Check sheet for the modelled part. Datum: model origin and axes. Units: mm. Face numbers are marked on the shaded views. A direction names the side the tool comes from. Give positions to 0.01 mm unless a question says otherwise; leave off trailing zeros. Answer as CSV lines item,"result". Start each with the question number.
(1) Section check A-A on x = 41.2. State how many separate pieces and enclosed holes the cut face has, plus the area to 3 significant figures.
(2) Material ranges on line 1 (X direction, y = -13.04, z = 2.6); line 2 (X direction, y = -12.7, z = 3.75); line 3 (Y direction, x = 41.2, z = 1.9), recorded low to high. Write a range as from..to.
(3) Access from +Z, -Z, +X, -X, +Y, -Y to the whole of each face (thin tool, end or side, straight path). Record for the marked faces 1 and 2.
(4) Gauge pin test, flat end, axial feed: pin 1 Ø5.5 at (x, y) = (41.5, -12.5) entering from +Z. Record the tip position at first contact, or that the pin passes through.
(5) Release check for a two-part mould opening along X. For the marked faces 3 and 4 record: pulls with the +X half, pulls with the -X half, needs draft (parallel to the pull), parting line crosses it, or undercut.
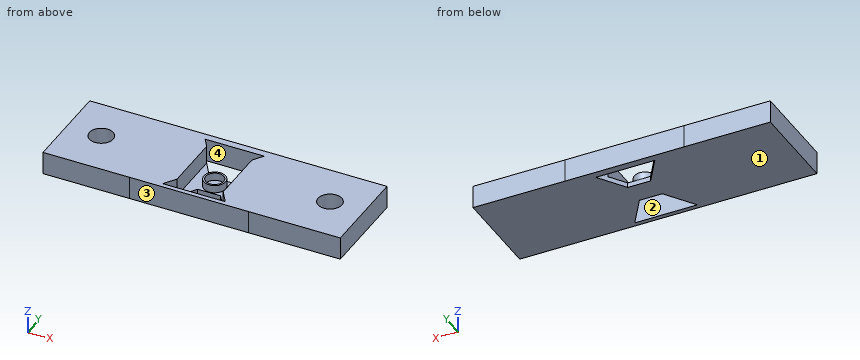
from build123d import *

# Parameters (mm, degrees)
BOX_W             = 33
BOX_H             = 2
BOX_DEPTH         = 6.35
CYLINDER001_R     = 3.302
CYLINDER001_DEPTH = 10
BOX002_W          = 12.7
BOX002_H          = 16.7
BOX002_DEPTH      = 17
CYLINDER_R        = 3.302
CYLINDER_DEPTH    = 10
EXTRUDE_DEPTH     = 6.35
CYLINDER003_R     = 2.5
CYLINDER003_DEPTH = 16
CYLINDER002_R     = 3
CYLINDER002_DEPTH = 3.5
BOX001_W          = 33
BOX001_H          = 1.25
BOX001_DEPTH      = 6.35


with BuildPart() as support1:
    # Box → Box (new body)
    with BuildSketch(Plane(origin=(24, -2.35, 0), x_dir=(1, 0, 0), z_dir=(0, 0, 1))):
        with Locations((16.5, 1)):
            Rectangle(BOX_W, BOX_H)
    extrude(amount=BOX_DEPTH)


with BuildPart() as hole2:
    # Cylinder001 → Cylinder001 (new body)
    with BuildSketch(Plane(origin=(73.025, -12.7, 1e-05), x_dir=(1, 0, 0), z_dir=(0, 0, 1))):
        Circle(CYLINDER001_R)
    extrude(amount=CYLINDER001_DEPTH)


with BuildPart() as thinner:
    # Box002 → Box002 (new body)
    with BuildSketch(Plane(origin=(34.85, -21.35, 1.35), x_dir=(1, 0, 0), z_dir=(0, 0, 1))):
        with Locations((6.35, 8.35)):
            Rectangle(BOX002_W, BOX002_H)
    extrude(amount=BOX002_DEPTH)


with BuildPart() as fusion:
    # Cylinder → Cylinder (new body)
    with BuildSketch(Plane(origin=(9.525, -12.7, 1e-05), x_dir=(1, 0, 0), z_dir=(0, 0, 1))):
        Circle(CYLINDER_R)
    extrude(amount=CYLINDER_DEPTH)

    # Fusion: union Hole2, Thinner
    add(hole2.part)
    add(thinner.part)


with BuildPart() as cut:
    with BuildSketch(Plane(origin=(41.275, -13.050916, 0), x_dir=(0, -1, 0), z_dir=(0, 0, -1))):
        with BuildLine():
            add(Edge.make_bspline(
                [(-12.7, 41.275), (-12.7, 9.525)],
                knots=[0, 0, 112.5, 112.5], degree=1))
            add(Edge.make_bspline(
                [(-12.7, 9.525), (-3.175, 3.175)],
                knots=[0, 0, 40.562452, 40.562452], degree=1))
            add(Edge.make_bspline(
                [(-3.175, 3.175), (-3.175, -3.175)],
                knots=[0, 0, 22.5, 22.5], degree=1))
            add(Edge.make_bspline(
                [(-3.175, -3.175), (-12.7, -9.525)],
                knots=[0, 0, 40.562452, 40.562452], degree=1))
            add(Edge.make_bspline(
                [(-12.7, -9.525), (-12.7, -41.275)],
                knots=[0, 0, 112.5, 112.5], degree=1))
            add(Edge.make_bspline(
                [(-12.7, -41.275), (12.7, -41.275)],
                knots=[0, 0, 90, 90], degree=1))
            add(Edge.make_bspline(
                [(12.7, -41.275), (12.7, -9.525)],
                knots=[0, 0, 112.5, 112.5], degree=1))
            add(Edge.make_bspline(
                [(12.7, -9.525), (3.175, -3.175)],
                knots=[0, 0, 40.562452, 40.562452], degree=1))
            add(Edge.make_bspline(
                [(3.175, -3.175), (3.175, 3.175)],
                knots=[0, 0, 22.5, 22.5], degree=1))
            add(Edge.make_bspline(
                [(3.175, 3.175), (12.7, 9.525)],
                knots=[0, 0, 40.562452, 40.562452], degree=1))
            add(Edge.make_bspline(
                [(12.7, 9.525), (12.7, 41.275)],
                knots=[0, 0, 112.5, 112.5], degree=1))
            add(Edge.make_bspline(
                [(12.7, 41.275), (-12.7, 41.275)],
                knots=[0, 0, 90, 90], degree=1))
        make_face()
    extrude(amount=-EXTRUDE_DEPTH)

    # Cut: cut Fusion
    add(fusion.part, mode=Mode.SUBTRACT)


with BuildPart() as cylinder001:
    # Cylinder003 → Cylinder003 (new body)
    with BuildSketch(Plane(origin=(41.2, -13.04, 0), x_dir=(1, 0, 0), z_dir=(0, 0, 1))):
        Circle(CYLINDER003_R)
    extrude(amount=CYLINDER003_DEPTH)


with BuildPart() as cut001:
    # Cylinder002 → Cylinder002 (new body)
    with BuildSketch(Plane(origin=(41.2, -13.04, 0), x_dir=(1, 0, 0), z_dir=(0, 0, 1))):
        Circle(CYLINDER002_R)
    extrude(amount=CYLINDER002_DEPTH)

    # Cut001: cut Cylinder001
    add(cylinder001.part, mode=Mode.SUBTRACT)


with BuildPart() as fusion001:
    # Box001 → Box001 (new body)
    with BuildSketch(Plane(origin=(24, -25.753, 0), x_dir=(1, 0, 0), z_dir=(0, 0, 1))):
        with Locations((16.5, 0.625)):
            Rectangle(BOX001_W, BOX001_H)
    extrude(amount=BOX001_DEPTH)

    # Fusion001: union Support1, Cut, Cut001
    add(support1.part)
    add(cut.part)
    add(cut001.part)


solid = fusion001.part
Working result:
1,separate pieces,"3"
1,enclosed holes,"0"
1,area,"31.4 mm^2"
2,line 1,"x = 0..6.24, 12.81..34.85, 38.2..38.7, 43.7..44.2, 47.55..69.74, 76.31..82.55"
2,line 2,"x = 0..6.22, 12.83..34.85, 47.55..69.72, 76.33..82.55"
2,line 3,"y = -25.75..-24.5, -16.04..-15.54, -10.54..-10.04, -2.35..-0.35"
3,face 1,"-Z, +X, -X, +Y, -Y"
3,face 2,"+Z, -Z"
4,pin 1,"stops at z = 3.5"
5,face 3,"needs draft"
5,face 4,"undercut"
